Verification items for the finished model (mm, model axes). Give positions to 0.01 mm unless a question says otherwise; leave off trailing zeros. Write each loop counter-clockwise with the first axis right and the second up, starting at its lowest first coordinate (ties: lowest second). Pieces come first, ordered by that corner, then holes. Notation, with made-up numbers: (71, 3) - (83, 3) arc R27 cw to (83, 39) - close; hole circle Ø6 at (40, 34.5). An arc over 180 degrees is marked (long way). Put each result on its own line as item: value.
from build123d import *

# Parameters (mm, degrees)
BOSS_EXTRUDE1_DEPTH = 2.921


with BuildPart() as part:
    # Sketch2 → Boss-Extrude1 (new body)
    with BuildSketch(Plane(origin=(0, 0, 0), x_dir=(1, 0, 0), z_dir=(0, 1, 0))):
        with BuildLine():
            Line((35.179, 0), (50.8, 0))
            ThreePointArc((50.8, 0), (39.252334483, 29.06354477), (12.319, 44.958))
            Line((12.319, 44.958), (0, 44.958))
            Line((0, 44.958), (0, 35.306))
            Line((0, 35.306), (-2.921, 35.306))
            Line((-2.921, 35.306), (-2.921, 9.652))
            Line((-2.921, 9.652), (0, 9.652))
            Line((0, 9.652), (0, 0))
            Line((0, 0), (22.479, 0))
            Line((22.479, 0), (22.479, -2.921))
            Line((22.479, -2.921), (35.179, -2.921))
            Line((35.179, -2.921), (35.179, 0))
        make_face()
    extrude(amount=BOSS_EXTRUDE1_DEPTH)


solid = part.part
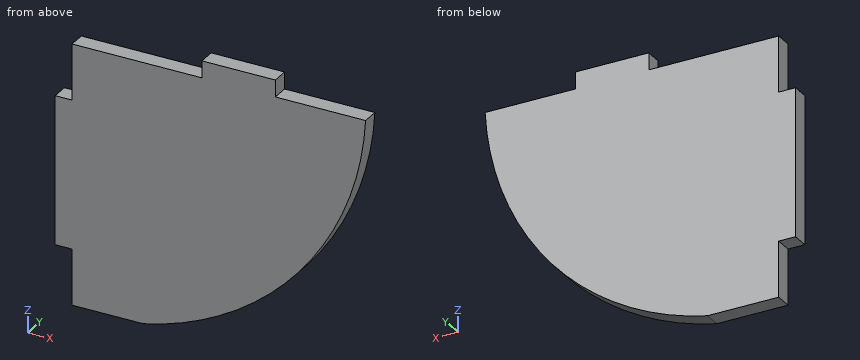
Q1. Section check A-A, the plane y = 0.9. Record the cut outline in (x, z), plus the area to 3 significant figures.
Answers follow:
outline: (-2.92, -35.31) - (0, -35.31) - (0, -44.96) - (12.32, -44.96) arc R48.29 ccw to (50.8, 0) - (35.18, 0) - (35.18, 2.92) - (22.48, 2.92) - (22.48, 0) - (0, 0) - (0, -9.65) - (-2.92, -9.65) - close
area: 1,940 mm2
Q2. Scan lines: line 1 along Z through (x, y) = (11, 0.35); line 2 along X through (y, z) = (0.75, -5.5); line 3 along X through (y, z) = (0.75, -19.5). Record each from-to range of solid material in increasing order.
Answers follow:
line 1: z = -44.96 to 0
line 2: x = 0 to 50.22
line 3: x = -2.92 to 45.64
Q3. Go/stop test with flat-tipped pins: pin 1 Ø0.9 at (y, z) = (1, 1.5) entering from -X; pin 2 Ø1.5 at (y, z) = (2, -41.5) entering from -X; pin 3 Ø1.5 at (x, y) = (-1, 1) entering from +Z. Record where each tip stops, or that it passes through.
Answers follow:
pin 1: stops at x = 22.48
pin 2: stops at x = 0
pin 3: stops at z = -9.65
Q4. Section check B-B, the plane x = 7. Record the cut outline in (y, z), plus the area to 3 significant figures.
Answers follow:
outline: (0, -44.96) - (2.92, -44.96) - (2.92, 0) - (0, 0) - close
area: 131 mm2
Q5. Section check C-C, the plane z = -8. Record the cut outline in (x, y), plus the area to 3 significant figures.
Answers follow:
outline: (0, 0) - (49.74, 0) - (49.74, 2.92) - (0, 2.92) - close
area: 145 mm2
